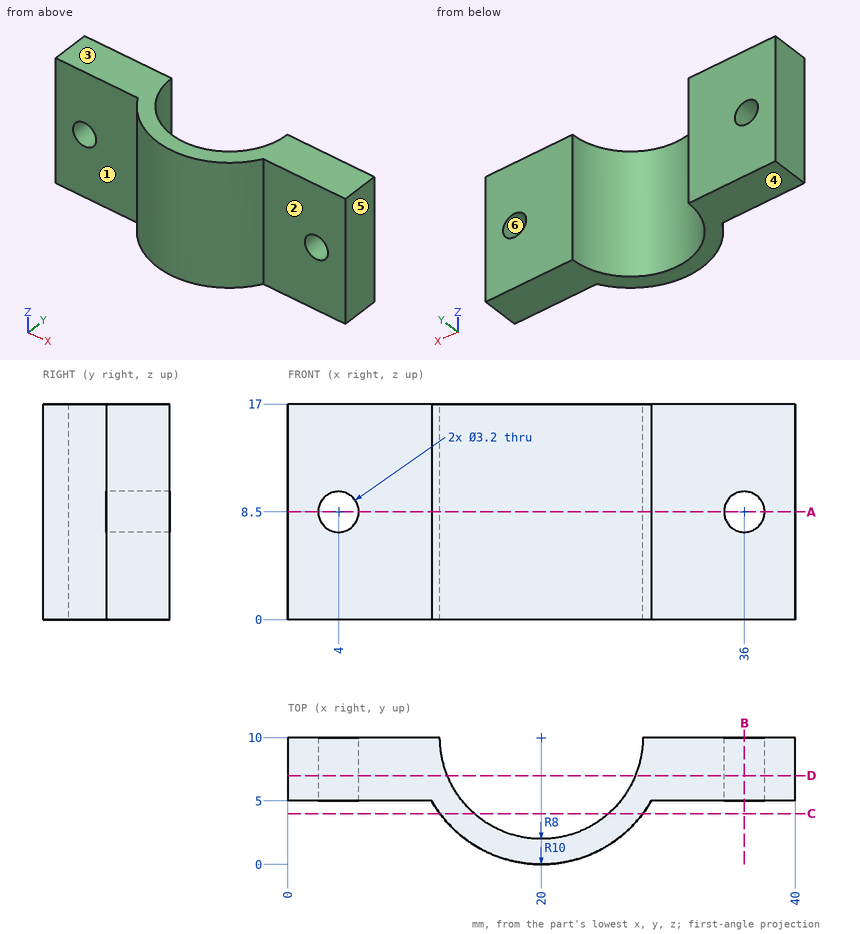
Verification items for this drawing (mm, ordinates from the low corner). A direction names the side the tool comes from. Round coordinates to 2 decimals unless told otherwise and drop trailing zeros. Write each loop counter-clockwise with the first axis right and the second up, starting at its lowest first coordinate (ties: lowest second). Pieces come first, ordered by that corner, then holes. Notation, with made-up numbers: M 69.5,79 L 83.5,79 A36 cw 83.5,115 Z; hole C -0.75,88 d3. An arc over 180 degrees is marked long. Write item = value, one per line. Start each with the question number.
1. Tool access check on the marked faces 1, 2 and 3. Record the directions out of +Z, -Z, +X, -X, +Y, -Y that give a thin tool (end or side, any length) a straight path to the whole face; none if there is none.
2. Section check B-B, the plane x = 36. Record the cut outline in (y, z).
3. Release check for a two-part mould opening along Z. For the marked faces 4, 5 and 6 record: pulls with the +Z half, pulls with the -Z half, needs draft (parallel to the pull), parting line crosses it, or undercut.
4. Section check C-C, the plane y = 4. Record the cut outline in (x, z), then the cut area to 3 significant figures.
5. Gauge pin test, flat ends, axial feed: pin 1 (1 mm diameter, centred on x = 32, z = 5.5, fed in from -Y); pin 2 (2.5 mm diameter, centred on x = 4, z = 8.5, fed in from +Y); pin 3 (9 mm diameter, centred on x = 7, z = 8.5, fed in from -Y); pin 4 (6 mm diameter, centred on x = 22.5, z = 4, fed in from +Y). Record the tip position at first contact, or that the pin passes through.
6. Scan lines: line 1 (Z direction, x = 4, y = 8.3); line 2 (Y direction, x = 5, z = 6.5); line 3 (X direction, y = 5.25, z = 4.5). Record each from-to range of solid material in increasing order. Write a range as [from, to].
7. Section check D-D, the plane y = 7. Record the cut outline in (x, z), then the cut area to 3 significant figures.
8. Section check A-A, the plane z = 8.5. Record the cut outline in (x, y).
Results found:
q1.face_1 = +Z, -Z, -X, -Y
q1.face_2 = +Z, -Z, +X, -Y
q1.face_3 = +Z, +X, -X, +Y, -Y
q2.outline = M 5,0 L 10,0 L 10,6.9 L 5,6.9 Z; M 5,10.1 L 10,10.1 L 10,17 L 5,17 Z
q3.face_4 = pulls with the -Z half
q3.face_5 = needs draft
q3.face_6 = undercut
q4.outline = M 12,0 L 14.71,0 L 14.71,17 L 12,17 Z; M 25.29,0 L 28,0 L 28,17 L 25.29,17 Z
q4.area = 92.1 mm^2
q5.pin_1 = 5
q5.pin_2 = through
q5.pin_3 = 4.73
q5.pin_4 = 4.19
q6.line_1 = [0, 6.9], [10.1, 17]
q6.line_2 = [5, 10]
q6.line_3 = [0, 13.56], [26.44, 40]
q7.outline = M 0,0 L 12.58,0 L 12.58,17 L 0,17 Z; M 27.42,0 L 40,0 L 40,17 L 27.42,17 Z; hole C 4,8.5 d3.2; hole C 36,8.5 d3.2
q7.area = 412 mm^2
q8.outline = M 0,5 L 2.4,5 L 2.4,10 L 0,10 Z; M 5.6,5 L 11.34,5 A10 ccw 28.66,5 L 34.4,5 L 34.4,10 L 28,10 A8 cw 12,10 L 5.6,10 Z; M 37.6,5 L 40,5 L 40,10 L 37.6,10 Z
